Design review of the part built by this model. Coordinates are the model's own, in mm. A direction names the side the tool comes from. Give positions to 0.01 mm unless a question says otherwise; leave off trailing zeros. Order: outer loops, then holes, each group sorted by start corner. A loop starts at its lowest first (then second) coordinate and runs counter-clockwise, first axis right, second up. Notation, with made-up numbers: (-22.5, 57.25) -> (1.5, 57.25) arc R15 ccw to (1.5, 82.25) -> close; hole circle Ø11 at (9.25, -24). An arc over 180 degrees is marked (long way). Return JSON: item names as keys, results as strings.
```python
from build123d import *


with BuildPart() as part:
    # Эскиз1 → Повернуть1 (revolve)
    with BuildSketch(Plane(origin=(0, 0, 0), x_dir=(0, 0, -1), z_dir=(1, 0, 0)), mode=Mode.PRIVATE) as revolve_1_sk:
        Polygon((-0.3, 0.1), (-0.3, 1.8), (0, 1.8), (0, 0), (-0.2, 0), align=None)
        Polygon((-0.65, 1.8), (-0.3, 1.8), (0, 1.8), (0, 2.2), (-0.625, 2.2), (-0.75, 2.2), (-0.75, 1.9), align=None)
        with BuildLine():
            Line((-0.625, 2.2), (0, 2.2))
            Line((0, 2.2), (0, 10.3))
            Line((0, 10.3), (-0.4, 10.3))
            Line((-0.4, 10.3), (-0.425, 10.3))
            ThreePointArc((-0.425, 10.3), (-0.566421356, 10.241421356), (-0.625, 10.1))
            Line((-0.625, 10.1), (-0.625, 2.2))
        make_face()
        with BuildLine():
            Line((-0.4, 10.3), (0, 10.3))
            Line((0, 10.3), (0, 11.8))
            Line((0, 11.8), (-0.03, 11.8))
            ThreePointArc((-0.03, 11.8), (-0.291629509, 11.691629509), (-0.4, 11.43))
            Line((-0.4, 11.43), (-0.4, 10.3))
        make_face()
    revolve(revolve_1_sk.sketch.rotate(Axis((0, 0, 0), (0, 1, 0)), 180), axis=Axis((0, 0, 0), (0, 1, 0)))


solid = part.part
```
Item 1: Add section B-B (y = 4). Give the boundary of the cut face in (x, z) (3 decimals).
Result set:
{"outline": "circle Ø1.25 at (0, 0)"}
Item 2: Machinability: for faces 1 (the face through (0.29, 2.05, -0.69)), 2 (the face through (-0.027, 6.095, 0.624)), which of the approach directions +Z, -Z, +X, -X, +Y, -Y give a long, thin tool a straight path to every point of the face, cutting with its end or side? Answer none if there is none.
Result set:
{"face 1": "+Y, -Y", "face 2": "+Y"}
Item 3: Add section A-A (y = 11). Give the boundary of the cut face in (x, z).
Result set:
{"outline": "circle Ø0.8 at (0, 0)"}
Item 4: Wall thickness on L1, parallel to Z at x = -0.05, y = 3.75; L2, parallel to X at y = 10.5, z = -0.3; L3, parallel to X at y = 7.75, z = -0.35: over which ranges is each line inside the solid? List them lowest first. Write a range as [from, to].
Result set:
{"L1": "z = [-0.62, 0.62]", "L2": "x = [-0.26, 0.26]", "L3": "x = [-0.52, 0.52]"}
